Work out the finished part from the listing and answer in its coordinate system (mm). Face numbers are marked on the shaded views. A direction names the side the tool comes from. Coordinates: 2 decimals unless noted, no trailing zeros. Order: outer loops, then holes, each group sorted by start corner. A loop starts at its lowest first (then second) coordinate and runs counter-clockwise, first axis right, second up.
1. Find the intervals of material crossed by probe 1 along Y at (x, z) = (-7.5, 4.4); probe 2 along X at (y, z) = (7.75, 4.05); probe 3 along X at (y, z) = (6, 1.3), in increasing order.
2. A tool of negligible diameter and unlimited length cuts with its end or side. For the marked faces 4 and 5, from which of +Z, -Z, +X, -X, +Y, -Y can it reach the whole face along a straight path? Write none if from no direction.
3. Flat-ended cylindrical pins translate along their axes: pin 1 Ø6 at (x, y) = (-6, 5.5) entering from +Z; pin 2 Ø2.5 at (x, y) = (-4.5, -5.5) entering from +Z. Find the tip coordinate at first contact, or state that the pin passes through.
4. The part is cut by section C-C, the plane z = 1.65. Give the vertices of the cut face in (x, y), then the cut area to 3 significant figures.
5. The part is cut by section B-B, the plane x = 0. Give the vertices of the cut face in (y, z), then the cut area to 3 significant figures.
6. The part is cut by section D-D, the plane x = -7. Give the vertices of the cut face in (y, z).
7. Determine the mould class of the marked faces 1, 2 and 3 for opening direction X: +X half, -X half, draft (parallel to the pull), parting line (faces both ways), or undercut.
8. The part is cut by section A-A, the plane y = 0. Give the vertices of the cut face in (x, z).
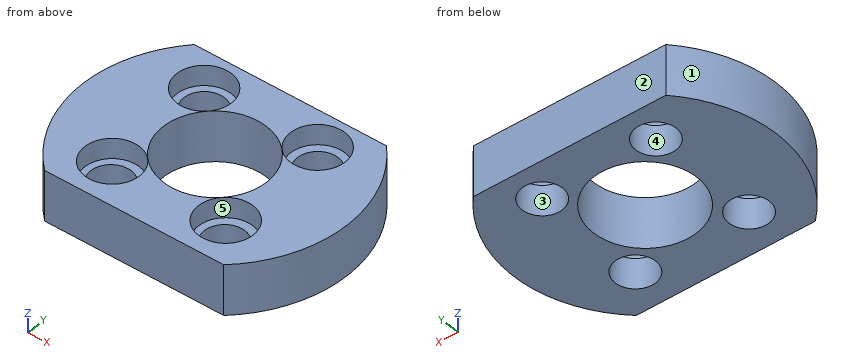
```python
from build123d import *

# Parameters (mm, degrees)
F0_R     = 2
F0_R_2   = 5.1
F1_DEPTH = 5
F2_R     = 2.7
F2_R_2   = 2
F3_DEPTH = 2


with BuildPart() as f1:
    # F0 (on Top) → F1 (new body)
    with BuildSketch(Plane.XY):
        with BuildLine():
            Line((-8.744989, -9.619), (8.744989, -9.619))
            ThreePointArc((8.744989, -9.619), (12.99212, -0.452563), (9.39311, 8.987185))
            Line((9.39311, 8.987185), (-9.39311, 8.987185))
            ThreePointArc((-9.39311, 8.987185), (-12.99212, -0.452563), (-8.744989, -9.619))
        make_face()
        with Locations((-5.553092, -5.619)):
            Circle(F0_R, mode=Mode.SUBTRACT)
        with Locations((5.553092, -5.619)):
            Circle(F0_R, mode=Mode.SUBTRACT)
        with Locations((-5.553092, 5.487185)):
            Circle(F0_R, mode=Mode.SUBTRACT)
        Circle(F0_R_2, mode=Mode.SUBTRACT)
        with Locations((5.553092, 5.487185)):
            Circle(F0_R, mode=Mode.SUBTRACT)
    extrude(amount=F1_DEPTH)

    # F2 (on face) → F3 (cut)
    with BuildSketch(Plane.XY.offset(5)):
        with Locations((-5.553092, 5.487185)):
            Circle(F2_R)
        with Locations((-5.553092, 5.487185)):
            Circle(F2_R_2, mode=Mode.SUBTRACT)
        with Locations((5.487185, 5.553092)):
            Circle(F2_R)
        with Locations((5.553092, 5.487185)):
            Circle(F2_R_2, mode=Mode.SUBTRACT)
        with Locations((5.553092, -5.487185)):
            Circle(F2_R)
        with Locations((5.553092, -5.619)):
            Circle(F2_R_2, mode=Mode.SUBTRACT)
        with Locations((-5.487185, -5.553092)):
            Circle(F2_R)
        with Locations((-5.553092, -5.619)):
            Circle(F2_R_2, mode=Mode.SUBTRACT)
    extrude(amount=-F3_DEPTH, mode=Mode.SUBTRACT)


solid = f1.part
```
Geometry says:
1. probe 1: y = -9.62 to -7.35, -3.75 to 3.62, 7.36 to 8.99
1. probe 2: x = -10.44 to -7.03, -4.08 to 3.92, 7.06 to 10.44
1. probe 3: x = -11.53 to -7.49, -3.62 to 3.62, 7.49 to 11.53
2. face 4: +Z, -Z
2. face 5: +Z
3. pin 1: stops at z = 5
3. pin 2: stops at z = 3
4. outline: (-9.39, 8.99) arc R13 ccw to (-8.74, -9.62) - (8.74, -9.62) arc R13 ccw to (9.39, 8.99) - close; hole circle Ø4 at (-5.55, -5.62); hole circle Ø4 at (-5.55, 5.49); hole circle Ø10.2 at (0, 0); hole circle Ø4 at (5.55, -5.62); hole circle Ø4 at (5.55, 5.49)
4. area: 306 mm2
5. outline: (-9.62, 0) - (-5.1, 0) - (-5.1, 5) - (-9.62, 5) - close; (5.1, 0) - (8.99, 0) - (8.99, 5) - (5.1, 5) - close
5. area: 42.0 mm2
6. outline: (-9.62, 0) - (-7, 0) - (-7, 3) - (-7.79, 3) - (-7.79, 5) - (-9.62, 5) - close; (-4.24, 0) - (4.11, 0) - (4.11, 3) - (3.21, 3) - (3.21, 5) - (-3.32, 5) - (-3.32, 3) - (-4.24, 3) - close; (6.87, 0) - (8.99, 0) - (8.99, 5) - (7.77, 5) - (7.77, 3) - (6.87, 3) - close
7. face 1: -X half
7. face 2: draft
7. face 3: undercut
8. outline: (-13, 0) - (-5.1, 0) - (-5.1, 5) - (-13, 5) - close; (5.1, 0) - (13, 0) - (13, 5) - (5.1, 5) - close
